```python
from build123d import *

# Parameters (mm, degrees)
BOSS_EXTRUDE1_DEPTH = 5
SKETCH8_R           = 9
BOSS_EXTRUDE3_DEPTH = 5
CUT_EXTRUDE1_REACH  = 53.228
SKETCH12_R          = 1
CUT_EXTRUDE2_DEPTH  = 0.5
SKETCH13_R          = 5
BOSS_EXTRUDE5_DEPTH = 5
CUT_EXTRUDE3_REACH  = 53.955
SKETCH15_R          = 2.4
CUT_EXTRUDE4_REACH  = 53.228
SKETCH16_R          = 2.4


with BuildPart() as part:
    # Sketch1 → Boss-Extrude1 (new body)
    with BuildSketch(Plane(origin=(0, 0, 0), x_dir=(0.4985289035363021, -0.866873077410351, 0), z_dir=(0, 0, 1))):
        with BuildLine():
            ThreePointArc((8.899126574, -3.909046337), (10.510039278, -0.019959041), (8.899126574, 3.869128256))
            Line((8.899126574, 3.869128256), (-2.35642803, 24.179978159))
            ThreePointArc((-2.35642803, 24.179978159), (-9.345167797, 25.255857552), (-10.421047189, 18.267117784))
            Line((-10.421047189, 18.267117784), (0.353553391, -2.434608777))
            Line((0.353553391, -2.434608777), (0.353553391, -46.838046337))
            Line((0.353553391, -46.838046337), (8.899126574, -46.838046337))
            Line((8.899126574, -46.838046337), (8.899126574, -3.909046337))
        make_face()
    extrude(amount=BOSS_EXTRUDE1_DEPTH)

    # Sketch8 → Boss-Extrude3 (add)
    with BuildSketch(Plane(origin=(0, 0, 0), x_dir=(-1, 0, 0), z_dir=(0, 0, -1))):
        with Locations((25.293181008, -19.882635909)):
            Circle(SKETCH8_R)
    extrude(amount=-BOSS_EXTRUDE3_DEPTH)

    # Sketch11 → Cut-Extrude1 (cut, up to next)
    with BuildSketch(Plane(origin=(0, 0, 0), x_dir=(-1, 0, 0), z_dir=(0, 0, -1)), mode=Mode.PRIVATE) as cut_extrude1_sk1:
        Polygon((26.471882365, -24.251922248), (29.662467347, -18.703934553), (24.114479652, -15.51334957), (20.923894669, -21.061337265), align=None)
    cut_extrude1_tool1 = extrude(cut_extrude1_sk1.sketch, amount=-CUT_EXTRUDE1_REACH, mode=Mode.PRIVATE) & part.part
    add(cut_extrude1_tool1.solids().sort_by_distance((-25.293181, -19.882636, 0))[0], mode=Mode.SUBTRACT)

    # Sketch12 → Cut-Extrude2 (cut)
    with BuildSketch(Plane(origin=(-24.825551359, -14.27689384, 0), x_dir=(0, 0, 1), z_dir=(-0.866873077410351, -0.49852890353630236, 0))):
        with Locations(Location((2.5, -4.626339983, 0), (0, 0, 270))):
            Circle(SKETCH12_R)
    extrude(amount=-CUT_EXTRUDE2_DEPTH, mode=Mode.SUBTRACT)

    # Sketch13 → Boss-Extrude5 (add)
    with BuildSketch(Plane(origin=(0, 0, 0), x_dir=(-1, 0, 0), z_dir=(0, 0, -1))):
        with Locations((-15.213151988, 16.118776732)):
            Circle(SKETCH13_R)
    extrude(amount=BOSS_EXTRUDE5_DEPTH)

    # Sketch15 → Cut-Extrude3 (cut, up to next)
    with BuildSketch(Plane(origin=(0, 0, -5), x_dir=(-1, 0, 0), z_dir=(0, 0, -1)), mode=Mode.PRIVATE) as cut_extrude3_sk1:
        with Locations((-15.213151988, 16.118776732)):
            Circle(SKETCH15_R)
    cut_extrude3_tool1 = extrude(cut_extrude3_sk1.sketch, amount=-CUT_EXTRUDE3_REACH, mode=Mode.PRIVATE) & part.part
    add(cut_extrude3_tool1.solids().sort_by_distance((15.213152, 16.118777, -5))[0], mode=Mode.SUBTRACT)

    # Sketch16 → Cut-Extrude4 (cut, up to next)
    with BuildSketch(Plane(origin=(0, 0, 0), x_dir=(-1, 0, 0), z_dir=(0, 0, -1)), mode=Mode.PRIVATE) as cut_extrude4_sk1:
        with Locations((-2.480347433, -4.353018325)):
            Circle(SKETCH16_R)
    cut_extrude4_tool1 = extrude(cut_extrude4_sk1.sketch, amount=-CUT_EXTRUDE4_REACH, mode=Mode.PRIVATE) & part.part
    add(cut_extrude4_tool1.solids().sort_by_distance((2.480347, -4.353018, 0))[0], mode=Mode.SUBTRACT)


solid = part.part
```
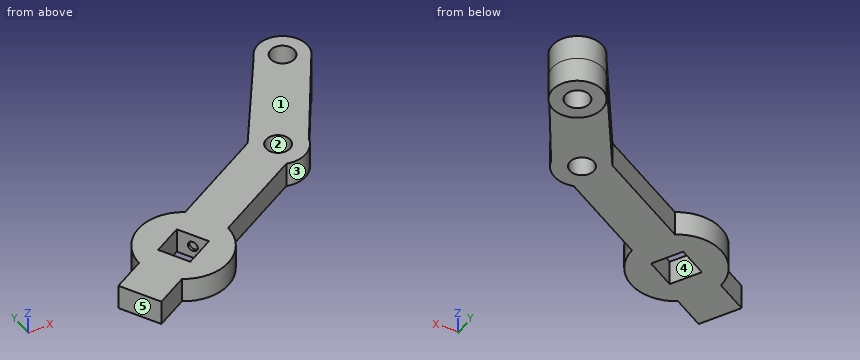
Geometry check sheet. Reference: the model listing, model coordinates, mm. Face numbers are marked on the shaded views. A direction names the side the tool comes from. Round coordinates to 2 decimals unless told otherwise and drop trailing zeros. Write each loop counter-clockwise with the first axis right and the second up, starting at its lowest first coordinate (ties: lowest second). Pieces come first, ordered by that corner, then holes. Notation, with made-up numbers: (81.5, 57.25) - (114.5, 57.25) arc R19 ccw to (114.5, 92.25) - close; hole circle Ø3 at (-11, -30). An arc over 180 degrees is marked (long way). Write each question's results on one line, items separated by ' | '.
(1) Sectioned sample at A-A, the plane x = 16. Enter the section's corners in (y, z).
Computed:
outline: (7.82, 0) - (11.18, 0) - (11.18, -5) - (13.85, -5) - (13.85, 5) - (7.82, 5) - close; (18.39, -5) - (21.06, -5) - (21.06, 5) - (18.39, 5) - close
(2) Sectioned sample at D-D, the plane y = -9. Enter the section's corners in (x, z), plus the area to 3 significant figures.
Computed:
outline: (-14.94, 0) - (5.42, 0) - (5.42, 5) - (-14.94, 5) - close | area: 102 mm^2
(3) Sectioned sample at C-C, the plane z = -1. Enter the section's corners in (x, y), plus the area to 3 significant figures.
Computed:
outline: circle Ø10 at (15.21, 16.12); hole circle Ø4.8 at (15.21, 16.12) | area: 60.4 mm^2
(4) Sectioned sample at B-B, the plane x = -27.5. Enter the section's corners in (y, z), plus the area to 3 significant figures.
Computed:
outline: (-28.61, 0) - (-22.46, 0) - (-22.46, 5) - (-28.61, 5) - close; (-17.46, 0) - (-11.16, 0) - (-11.16, 5) - (-17.46, 5) - close | area: 62.2 mm^2
(5) Depth check by flat-ended pin: pin 1 Ø5 at (x, z) = (-32, 2) entering from -Y; pin 2 Ø2 at (y, z) = (-17, 3.5) entering from +X; pin 3 Ø24.5 at (x, y) = (-22, -11.5) entering from -Z; pin 4 Ø6 at (x, y) = (15.21, 16.12) entering from -Z. Enter the tip coordinate at first touch or a pass-through.
Computed:
pin 1: stops at y = -30.11 | pin 2: stops at x = -9.97 | pin 3: stops at z = 0 | pin 4: stops at z = -5
(6) Draft check along Y on the marked faces 1, 2 and 3. Enter one of: pulls with the +Y half, pulls with the -Y half, needs draft (parallel to the pull), parting line crosses it, or undercut.
Computed:
face 1: needs draft | face 2: undercut | face 3: pulls with the -Y half
(7) Set-up check for the marked faces 4 and 5: record each of +Z, -Z, +X, -X, +Y, -Y from which the full face is reachable in a straight line by a thin tool's end or side.
Computed:
face 4: +Z, -Z | face 5: +Z, -Z, -X, -Y
(8) Thickness scan on probe 1 along Z at (x, y) = (-9.5, -6.5); probe 2 along Y at (x, z) = (-25, 0.5); probe 3 along Y at (x, z) = (-21, 2). Record the ranges inside material, lowest first. Write a range as from..to.
Computed:
probe 1: z = 0..5 | probe 2: y = -28.88..-23.41, -16.02..-10.89 | probe 3: y = -27.79..-21.11, -20.93..-11.97
